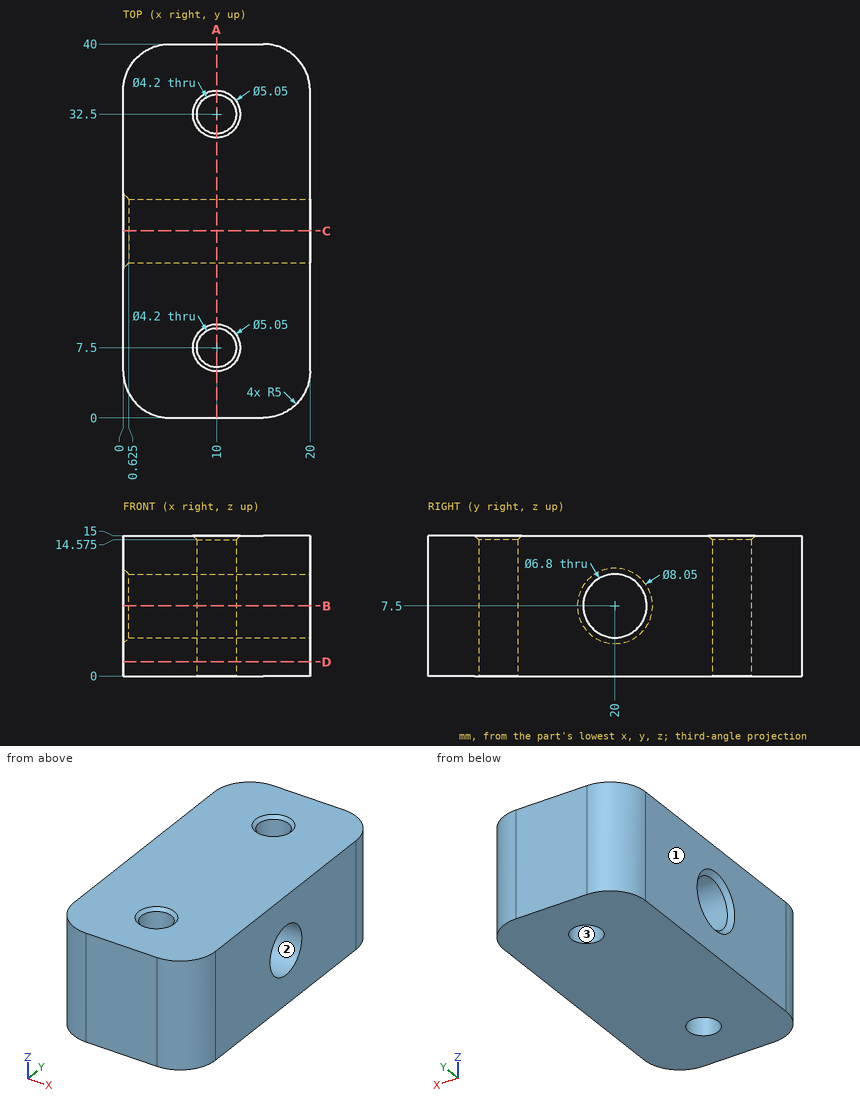
Can you work these out from the drawing? Everything is in mm from the part's minimum corner. Round coordinates to 2 decimals unless told otherwise and drop trailing zeros. Loops run counter-clockwise (first coordinate to the right, second up) from the corner with the lowest first, then second, coordinate; pieces in that order, holes last.
1. If I drill on line 1 along Y through (x, z) = (10, 7.5); line 2 along X through (y, z) = (7.5, 6.25); line 3 along Y through (x, z) = (11, 8.5), over which ranges is the centre line in solid material (lowest first)?
Answer list:
line 1: y = 0 to 5.4, 9.6 to 16.6, 23.4 to 30.4, 34.6 to 40
line 2: x = 0 to 7.9, 12.1 to 20
line 3: y = 0 to 5.65, 9.35 to 16.75, 23.25 to 30.65, 34.35 to 40
2. We'd pull the mould along X, two halves only. Please class the marked faces 1, 2 and 3: +X half, -X half, draft (parallel to the pull), parting line (faces both ways), or undercut.
Answer list:
face 1: -X half
face 2: draft
face 3: undercut
3. If we section it at D-D on z = 1.5: Write out the boundary of the cut face in (x, y), plus the area to 3 significant figures.
Answer list:
outline: (0, 5) arc R5 ccw to (5, 0) - (15, 0) arc R5 ccw to (20, 5) - (20, 35) arc R5 ccw to (15, 40) - (5, 40) arc R5 ccw to (0, 35) - close; hole circle Ø4.2 at (10, 7.5); hole circle Ø4.2 at (10, 32.5)
area: 751 mm2
4. For P1, Ø8, axis at y = 20, z = 7.5, coming from the -X side (3 decimals); P2, Ø1, axis at x = 17.5, z = 4, coming from the +Y side; P3, Ø3.5, axis at x = 10, y = 7.5, coming from the -Z side, each with a flat end and sliding along its axis, tell me the tip position at first contact or that it passes through.
Answer list:
P1: stops at x = 0.025
P2: stops at y = 39.58
P3: passes through
5. If we section it at C-C on y = 20: Write out the boundary of the cut face in (x, z) (3 decimals), plus the area to 3 significant figures.
Answer list:
outline: (0, 0) - (20, 0) - (20, 4.1) - (0.625, 4.1) - (0, 3.475) - close; (0, 11.525) - (0.625, 10.9) - (20, 10.9) - (20, 15) - (0, 15) - close
area: 164 mm2
6. If we section it at A-A on x = 10: Write out the boundary of the cut face in (y, z) (3 decimals), plus the area to 3 significant figures.
Answer list:
outline: (0, 0) - (5.4, 0) - (5.4, 14.575) - (4.975, 15) - (0, 15) - close; (9.6, 0) - (30.4, 0) - (30.4, 14.575) - (29.975, 15) - (10.025, 15) - (9.6, 14.575) - close; (34.6, 0) - (40, 0) - (40, 15) - (35.025, 15) - (34.6, 14.575) - close; hole circle Ø6.8 at (20, 7.5)
area: 437 mm2
7. If we section it at B-B on z = 7.5: Write out the boundary of the cut face in (x, y) (3 decimals), plus the area to 3 significant figures.
Answer list:
outline: (0, 5) arc R5 ccw to (5, 0) - (15, 0) arc R5 ccw to (20, 5) - (20, 16.6) - (0.625, 16.6) - (0, 15.975) - close; (0, 24.025) - (0.625, 23.4) - (20, 23.4) - (20, 35) arc R5 ccw to (15, 40) - (5, 40) arc R5 ccw to (0, 35) - close; hole circle Ø4.2 at (10, 7.5); hole circle Ø4.2 at (10, 32.5)
area: 614 mm2
